Verification items for the finished model (mm, model axes). Face numbers are marked on the shaded views. A direction names the side the tool comes from. Give positions to 0.01 mm unless a question says otherwise; leave off trailing zeros. Write each loop counter-clockwise with the first axis right and the second up, starting at its lowest first coordinate (ties: lowest second). Pieces come first, ordered by that corner, then holes. Notation, with made-up numbers: M 42.25,-4.75 L 59.25,-4.75 A23 ccw 59.25,11.25 Z; hole C 78,75.5 d1. An arc over 180 degrees is marked long. Answer as a JSON object with one key per item and string values.
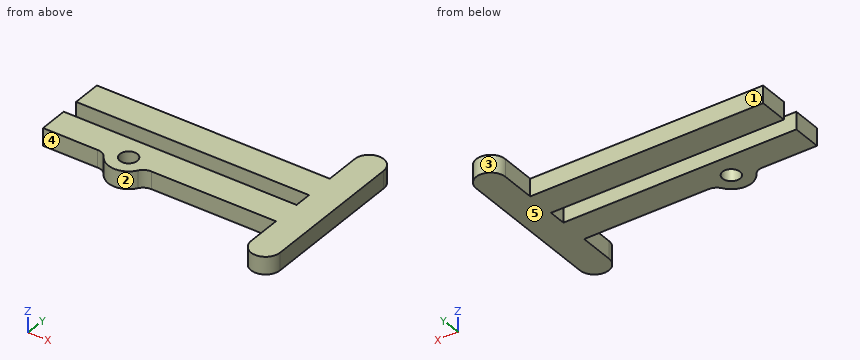
```python
from build123d import *

# Parameters (mm, degrees)
EXTRUDE_1_DEPTH     = 3
SKETCH_2_R          = 3.5
EXTRUDE_2_DEPTH     = 3
SKETCH_3_R          = 1.5
CUT_EXTRUDE_1_DEPTH = 48.689097286
EXTRUDE_3_DEPTH     = 3
FILLET_1_R          = 2


with BuildPart() as part:
    # 草图1 → 凸台-拉伸1 (new body)
    with BuildSketch(Plane.XY):
        Polygon((-45, 0), (0, 0), (0, -13), (-45, -13), (-45, -8), (-5, -8), (-5, -5), (-45, -5), align=None)
    extrude(amount=EXTRUDE_1_DEPTH)

    # 草图2 → 凸台-拉伸2 (add)
    with BuildSketch(Plane.XY.offset(3)):
        with Locations((-31, -12)):
            Circle(SKETCH_2_R)
    extrude(amount=-EXTRUDE_2_DEPTH)

    # 草图3 → 切除-拉伸1 (cut, through all)
    with BuildSketch(Plane.XY.offset(3)):
        with Locations((-31, -12)):
            Circle(SKETCH_3_R)
    extrude(amount=-CUT_EXTRUDE_1_DEPTH, mode=Mode.SUBTRACT)

    # 草图4 → 凸台-拉伸3 (add)
    with BuildSketch(Plane.XY):
        with BuildLine():
            Line((0, 6), (0, -19))
            ThreePointArc((0, -19), (-2.5, -21.5), (-5, -19))
            Line((-5, -19), (-5, 6))
            ThreePointArc((-5, 6), (-2.5, 8.5), (0, 6))
        make_face()
    extrude(amount=EXTRUDE_3_DEPTH)

    # 圆角1
    fillet_1_edges = [part.edges().sort_by_distance(p)[0] for p in [
        (-34.354101966, -13, 1.5),
        (-27.645898034, -13, 1.5),
    ]]
    fillet(fillet_1_edges, radius=FILLET_1_R)


solid = part.part
```
1) Section check D-D on x = -16. Record the boundary of the cut face in (y, z), and give its area (3 significant figures).
Completed:
{"outline": "M -13,0 L -8,0 L -8,3 L -13,3 Z; M -5,0 L 0,0 L 0,3 L -5,3 Z", "area": "30.0 mm2"}
2) Section check B-B on x = -31.5. Record the boundary of the cut face in (y, z), and give its area (3 significant figures).
Completed:
{"outline": "M -15.46,0 L -13.41,0 L -13.41,3 L -15.46,3 Z; M -10.59,0 L -8,0 L -8,3 L -10.59,3 Z; M -5,0 L 0,0 L 0,3 L -5,3 Z", "area": "28.9 mm2"}
3) Thickness scan on L1, parallel to Y at x = -31, z = 2.25; L2, parallel to Y at x = -32, z = 0.65; L3, parallel to Y at x = -16, z = 2.25. Record the ranges inside material, lowest first.
Completed:
{"L1": "y = -15.5 to -13.5, -10.5 to -8, -5 to 0", "L2": "y = -15.35 to -13.12, -10.88 to -8, -5 to 0", "L3": "y = -13 to -8, -5 to 0"}
4) Access from +Z, -Z, +X, -X, +Y, -Y to the whole of each face (thin tool, end or side, straight path). Record for the marked faces 4 and 5.
Completed:
{"face 4": "+Z, -Z, -X, -Y", "face 5": "-Z, +X, -X, +Y, -Y"}
5) Release check for a two-part mould opening along X. For the marked faces 1, 2 and 3 record: pulls with the +X half, pulls with the -X half, needs draft (parallel to the pull), parting line crosses it, or undercut.
Completed:
{"face 1": "needs draft", "face 2": "undercut", "face 3": "parting line crosses it"}
6) Go/stop test with flat-tipped pins: pin 1 (1.5 mm diameter, centred on x = -18.5, z = 1.5, fed in from -Y); pin 2 (0.9 mm diameter, centred on y = -14.5, z = 1.5, fed in from -X); pin 3 (0.9 mm diameter, centred on x = -18, z = 1.5, fed in from +Y); pin 4 (1.8 mm diameter, centred on x = -31, y = -12, fed in from -Z). Record where each tip stops, or that it passes through.
Completed:
{"pin 1": "stops at y = -13", "pin 2": "stops at x = -33.84", "pin 3": "stops at y = 0", "pin 4": "passes through"}
7) Section check C-C on z = 2.35. Record the boundary of the cut face in (x, y), and give its area (3 significant figures).
Completed:
{"outline": "M -45,-13 L -35.61,-13 A2 cw -33.93,-13.91 A3.5 ccw -28.07,-13.91 A2 cw -26.39,-13 L -5,-13 L -5,-19 A2.5 ccw 0,-19 L 0,6 A2.5 ccw -5,6 L -5,0 L -45,0 L -45,-5 L -5,-5 L -5,-8 L -45,-8 Z; hole C -31,-12 d3", "area": "550 mm2"}
8) Section check A-A on y = -12. Record the boundary of the cut face in (x, z), and give its area (3 significant figures).
Completed:
{"outline": "M -45,0 L -32.5,0 L -32.5,3 L -45,3 Z; M -29.5,0 L 0,0 L 0,3 L -29.5,3 Z", "area": "126 mm2"}
